Part model, mm, in its own coordinate system. Face numbers are marked on the shaded views. A direction names the side the tool comes from. Give positions to 0.01 mm unless a question says otherwise; leave off trailing zeros. Order: outer loops, then holes, each group sorted by start corner. A loop starts at its lowest first (then second) coordinate and runs counter-clockwise, first axis right, second up.
1. Slice it at A-A on y = 0. List the corners of the cut face in (x, z), and give its area (3 significant figures).
2. Drop flat-ended pins along their axis: pin 1 Ø5 at (x, y) = (0, 0) entering from +Z; pin 2 Ø1.5 at (y, z) = (19, 1) entering from +X; pin 3 Ø1 at (y, z) = (-3, 2) entering from -X; pin 4 Ø1.5 at (x, z) = (-3.5, 3) entering from +Y. Give the stop position or say it passes through.
3. Mould opens along Y. For the marked faces 5, 6 and 7 say: +Y half, -Y half, draft (parallel to the pull), parting line (faces both ways), or undercut.
4. Probe line 1 (Y direction, x = 0, z = 1.35); line 2 (X direction, y = 10.5, z = 1.25); line 3 (Y direction, x = 1, z = 3.2). List the from-to ranges inside material, lowest first.
5. Slice it at C-C on y = 16. List the corners of the cut face in (x, z), and give its area (3 significant figures).
6. Which spindle directions (+Z, -Z, +X, -X, +Y, -Y) get a long thin tool onto all of the face, cutting with end or side? Do the marked faces 1, 2, 3 and 4. Say none if no direction does.
7. Slice it at B-B on z = 1.45. List the corners of the cut face in (x, y).
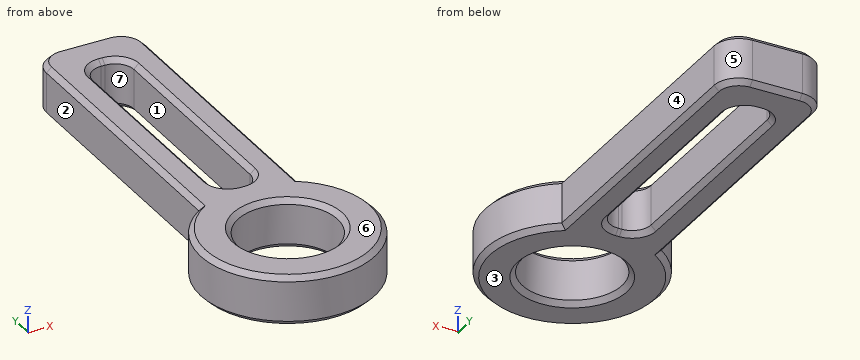
from build123d import *

# Parameters (mm, degrees)
BOX001001002_W     = 3.3
BOX001001002_H     = 20
BOX001001002_DEPTH = 10
FILLET001_R        = 1.5
BOX001001003_W     = 8
BOX001001003_H     = 25
BOX001001003_DEPTH = 4
FILLET002_R        = 2
CHAMFER002_SIZE    = 0.4
TUBE_R             = 7
TUBE_R_2           = 4
TUBE_DEPTH         = 4
CHAMFER001_SIZE    = 0.4


with BuildPart() as fillet001:
    # Box001001002 → Box001001002 (new body)
    with BuildSketch(Plane(origin=(-1.65, 7, 0), x_dir=(1, 0, 0), z_dir=(0, 0, 1))):
        with Locations((1.65, 10)):
            Rectangle(BOX001001002_W, BOX001001002_H)
    extrude(amount=BOX001001002_DEPTH)

    # Fillet001
    fillet001_edges = [fillet001.edges().sort_by_distance(p)[0] for p in [
        (-1.65, 7, 5),
        (-1.65, 27, 5),
        (1.65, 7, 5),
        (1.65, 27, 5),
    ]]
    fillet(fillet001_edges, radius=FILLET001_R)


with BuildPart() as chamfer002:
    # Box001001003 → Box001001003 (new body)
    with BuildSketch(Plane(origin=(-4, 5, 0), x_dir=(1, 0, 0), z_dir=(0, 0, 1))):
        with Locations((4, 12.5)):
            Rectangle(BOX001001003_W, BOX001001003_H)
    extrude(amount=BOX001001003_DEPTH)

    # Fillet002
    fillet002_edges = [chamfer002.edges().sort_by_distance(p)[0] for p in [
        (-4, 30, 2),
        (4, 30, 2),
    ]]
    fillet(fillet002_edges, radius=FILLET002_R)

    # Cut002008023012009006003002007003: cut Fillet001
    add(fillet001.part, mode=Mode.SUBTRACT)

    # Chamfer002
    chamfer002_edges = [chamfer002.edges().sort_by_distance(p)[0] for p in [
        (-4, 16.5, 4),
        (-4, 16.5, 0),
        (-3.414214, 29.414214, 4),
        (0, 5, 4),
        (0, 30, 4),
        (4, 16.5, 4),
        (3.414214, 29.414214, 4),
        (-1.21066, 7.43934, 4),
        (0, 7, 4),
        (1.21066, 7.43934, 4),
        (1.65, 17, 4),
        (1.21066, 26.56066, 4),
        (0, 27, 4),
        (-1.21066, 26.56066, 4),
        (-1.65, 17, 4),
        (0, 5, 0),
        (-3.414214, 29.414214, 0),
        (0, 30, 0),
        (4, 16.5, 0),
        (3.414214, 29.414214, 0),
        (-1.21066, 7.43934, 0),
        (0, 7, 0),
        (1.21066, 7.43934, 0),
        (1.65, 17, 0),
        (1.21066, 26.56066, 0),
        (0, 27, 0),
        (-1.21066, 26.56066, 0),
        (-1.65, 17, 0),
    ]]
    chamfer(chamfer002_edges, length=CHAMFER002_SIZE)


with BuildPart() as ptfe_tube_guide_arm_straight:
    # Tube → Tube (new body)
    with BuildSketch(Plane.XY):
        Circle(TUBE_R)
        Circle(TUBE_R_2, mode=Mode.SUBTRACT)
    extrude(amount=TUBE_DEPTH)

    # Chamfer001
    chamfer001_edges = [ptfe_tube_guide_arm_straight.edges().sort_by_distance(p)[0] for p in [
        (-7, 0, 4),
        (-7, 0, 0),
        (-4, 0, 4),
        (-4, 0, 0),
    ]]
    chamfer(chamfer001_edges, length=CHAMFER001_SIZE)

    # Fusion001: union Chamfer002
    add(chamfer002.part)


solid = ptfe_tube_guide_arm_straight.part
Data:
1. outline: (-7, 0.4) - (-6.6, 0) - (-4.4, 0) - (-4, 0.4) - (-4, 3.6) - (-4.4, 4) - (-6.6, 4) - (-7, 3.6) - close; (4, 0.4) - (4.4, 0) - (6.6, 0) - (7, 0.4) - (7, 3.6) - (6.6, 4) - (4.4, 4) - (4, 3.6) - close
1. area: 23.4 mm2
2. pin 1: passes through
2. pin 2: stops at x = 4
2. pin 3: stops at x = -6.54
2. pin 4: stops at y = 29.85
3. face 5: +Y half
3. face 6: draft
3. face 7: undercut
4. line 1: y = -7 to -4, 4 to 7, 27 to 30
4. line 2: x = -4 to -1.65, 1.65 to 4
4. line 3: y = -6.93 to -3.87, 3.87 to 7.26, 26.74 to 30
5. outline: (-4, 0.4) - (-3.6, 0) - (-2.05, 0) - (-1.65, 0.4) - (-1.65, 3.6) - (-2.05, 4) - (-3.6, 4) - (-4, 3.6) - close; (1.65, 0.4) - (2.05, 0) - (3.6, 0) - (4, 0.4) - (4, 3.6) - (3.6, 4) - (2.05, 4) - (1.65, 3.6) - close
5. area: 18.2 mm2
6. face 1: +Z, -Z
6. face 2: +Z, -Z, -X, +Y
6. face 3: -Z, +X, -X, +Y, -Y
6. face 4: +Z, -Z, +X, +Y
7. outline: (-4, 5.74) arc R7 ccw (long way) to (4, 5.74) - (4, 28) arc R2 ccw to (2, 30) - (-2, 30) arc R2 ccw to (-4, 28) - close; hole circle Ø8 at (0, 0); hole (-1.65, 8.5) arc R1.5 ccw to (-0.15, 7) - (0.15, 7) arc R1.5 ccw to (1.65, 8.5) - (1.65, 25.5) arc R1.5 ccw to (0.15, 27) - (-0.15, 27) arc R1.5 ccw to (-1.65, 25.5) - close
